```python
from build123d import *

# Parameters (mm, degrees)
F1_DEPTH = 50
F2_R     = 5
F3_DEPTH = 25
F4_R     = 5
F5_DEPTH = 25


with BuildPart() as f1:
    # F0 (on Front) → F1 (new body)
    with BuildSketch(Plane.XZ):
        with BuildLine():
            Line((-53.070944, 22.410468), (-53.070944, -36.589532))
            Line((-53.070944, -36.589532), (-47.070944, -36.589532))
            Line((-47.070944, -36.589532), (-47.070944, 22.410468))
            ThreePointArc((-47.070944, 22.410468), (-44.142012, 29.481535), (-37.070944, 32.410468))
            Line((-37.070944, 32.410468), (66.929056, 32.410468))
            Line((66.929056, 32.410468), (66.929056, 38.410468))
            Line((66.929056, 38.410468), (-37.070944, 38.410468))
            ThreePointArc((-37.070944, 38.410468), (-48.384652, 33.724176), (-53.070944, 22.410468))
        make_face()
    extrude(amount=F1_DEPTH)

    # F2 (on face) → F3 (cut)
    with BuildSketch(Plane.XY.offset(38.410468)):
        with Locations((-23.070944, -25)):
            Circle(F2_R)
        with Locations((36.929056, -25)):
            Circle(F2_R)
    extrude(amount=-F3_DEPTH, mode=Mode.SUBTRACT)

    # F4 (on face) → F5 (cut)
    with BuildSketch(Plane(origin=(-53.070944, 0, 0), x_dir=(0, -1, 0), z_dir=(-1, 0, 0))):
        with Locations((12.5, -1.589532)):
            Circle(F4_R)
        with Locations((37.5, -21.589532)):
            Circle(F4_R)
    extrude(amount=-F5_DEPTH, mode=Mode.SUBTRACT)


solid = f1.part
```
Source: CAD feature listing. Evaluate the final solid. Frame: model axes, mm. A direction names the side the tool comes from. Give positions to 0.01 mm unless a question says otherwise; leave off trailing zeros. Write each loop counter-clockwise with the first axis right and the second up, starting at its lowest first coordinate (ties: lowest second). Pieces come first, ordered by that corner, then holes.
1. Access query for faces 1 (the face through (14, -25, 32.41)), 2 (the face through (-50.113, -32.505, -21.37)). Directions: +Z, -Z, +X, -X, +Y, -Y. A direction counts if a zero-diameter tool reaches every point of the face in a straight line with its end or side. Return the directions, or none.
2. Material intervals for line 1 along X through (y, z) = (-33, 3.5); line 2 along Z through (x, y) = (-0.5, -44.5); line 3 along Z through (x, y) = (-49, -12), sorted ascending.
3. Section query C-C (z = -5). Return the cut outline in (x, y).
4. Section query B-B (y = -37.5). Return the cut outline in (x, z).
5. Section query D-D (z = 11). Return the cut outline in (x, y).
6. Section query A-A (y = -25). Return the cut outline in (x, z).
7. First-contact query: pin 1 (6 mm diameter, centred on x = -23.07, y = -25, fed in from -Z); pin 2 (4 mm diameter, centred on x = -23.5, y = -33.5, fed in from -Z); pin 3 (5 mm diameter, centred on y = -7, z = -23, fed in from +X); pin 4 (1.5 mm diameter, centred on y = -13.5, z = 24.5, fed in from -X). Flat tips, straight axial feed; report the tip coordinate or a pass-through.
8. Pull-direction query (Y, two-part tool) for faces 3 (the face through (-44.22, -24.65, 29.4)), 4 (the face through (-11, 0, 34)), 5 (the face through (-50.11, -17.27, -0.09)), 6 (the face through (41.548, -26.915, 35.452)); classes: +Y half, -Y half, draft (parallel to the pull), parting line (faces both ways), or undercut.
Output values:
1. face 1: -Z, +X, +Y, -Y
1. face 2: +X, -X
2. line 1: x = -53.07 to -47.07
2. line 2: z = 32.41 to 38.41
2. line 3: z = -36.59 to -6.56, 3.39 to 33.07
3. outline: (-53.07, -50) - (-47.07, -50) - (-47.07, -16.16) - (-53.07, -16.16) - close; (-53.07, -8.84) - (-47.07, -8.84) - (-47.07, 0) - (-53.07, 0) - close
4. outline: (-53.07, -36.59) - (-47.07, -36.59) - (-47.07, -26.59) - (-53.07, -26.59) - close; (-53.07, -16.59) - (-47.07, -16.59) - (-47.07, 22.41) arc R10 cw to (-37.07, 32.41) - (66.93, 32.41) - (66.93, 38.41) - (-37.07, 38.41) arc R16 ccw to (-53.07, 22.41) - close
5. outline: (-53.07, -50) - (-47.07, -50) - (-47.07, 0) - (-53.07, 0) - close
6. outline: (-53.07, -36.59) - (-47.07, -36.59) - (-47.07, 22.41) arc R10 cw to (-37.07, 32.41) - (-28.07, 32.41) - (-28.07, 38.41) - (-37.07, 38.41) arc R16 ccw to (-53.07, 22.41) - close; (-18.07, 32.41) - (31.93, 32.41) - (31.93, 38.41) - (-18.07, 38.41) - close; (41.93, 32.41) - (66.93, 32.41) - (66.93, 38.41) - (41.93, 38.41) - close
7. pin 1: passes through
7. pin 2: stops at z = 32.41
7. pin 3: stops at x = -47.07
7. pin 4: stops at x = -53.01
8. face 3: draft
8. face 4: +Y half
8. face 5: undercut
8. face 6: undercut
